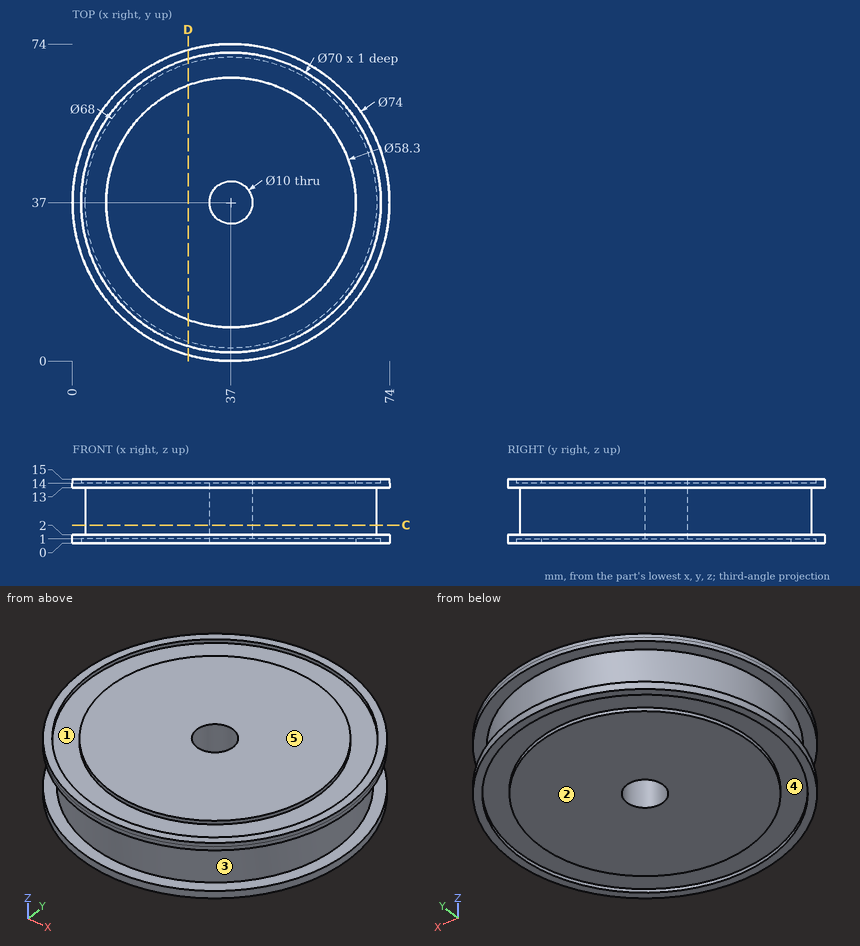
The figure shows three views and two pictorial views of one solid part (mm, origin at its lowest corner). Answer the questions. A direction names the side the tool comes from. Round coordinates to 2 decimals unless told otherwise and drop trailing zeros. Order: outer loops, then holes, each group sorted by start corner. A loop starts at its lowest first (then second) coordinate and runs counter-clockwise, first axis right, second up. Notation, with made-up numbers: M 4,73.5 L 54,73.5 A16 ccw 54,78.5 Z; hole C -22,39.25 d8. An arc over 180 degrees is marked long. Put each result on its own line as item: value. Start each with the question number.
Q1. Section D-D, the plane x = 27 is taken. Write down the section's boundary in (y, z), and give its area (3 significant figures).
Q2. For a pull along X with two mould halves and no side action, classify the marked faces 1, 2 and 3 as pulls with the +X half, pulls with the -X half, needs draft (parallel to the pull), parting line crosses it, or undercut.
Q3. Straight lines are drawn through the part: L1, parallel to Y at x = 37, z = 0.65; L2, parallel to Y at x = 37, z = 11; L3, parallel to Z at x = 67, y = 17. For each, find the intervals that lie inside material, in ascending order. Write a range as [from, to].
Q4. Flat-ended cylindrical pins translate along their axes: pin 1 (1.5 mm diameter, centred on x = 8.5, z = 6.5, fed in from -Y); pin 2 (2 mm diameter, centred on x = 20.5, z = 4.5, fed in from -Y); pin 3 (9 mm diameter, centred on x = 37, y = 37, fed in from +Z); pin 4 (3 mm diameter, centred on y = 36, z = 6, fed in from -X). Find the tip coordinate at first contact, or state that the pin passes through.
Q5. A tool of negligible diameter and unlimited length cuts with its end or side. For the marked faces 4 and 5, from which of +Z, -Z, +X, -X, +Y, -Y can it reach the whole face along a straight path? Write none if from no direction.
Q6. Section C-C, the plane z = 4.25 is taken. Write down the section's boundary in (x, y), and give its area (3 significant figures).
Findings below:
1. outline: M 1.38,0 L 3.46,0 L 3.46,1 L 9.62,1 L 9.62,0 L 64.38,0 L 64.38,1 L 70.54,1 L 70.54,0 L 72.62,0 L 72.62,2 L 69.5,2 L 69.5,13 L 72.62,13 L 72.62,15 L 70.54,15 L 70.54,14 L 64.38,14 L 64.38,15 L 9.62,15 L 9.62,14 L 3.46,14 L 3.46,15 L 1.38,15 L 1.38,13 L 4.5,13 L 4.5,2 L 1.38,2 Z
1. area: 975 mm^2
2. face 1: undercut
2. face 2: needs draft
2. face 3: parting line crosses it
3. L1: y = [0, 2], [7.85, 32], [42, 66.15], [72, 74]
3. L2: y = [3, 32], [42, 71]
3. L3: z = [0, 2], [13, 15]
4. pin 1: stops at y = 17.35
4. pin 2: stops at y = 6.74
4. pin 3: passes through
4. pin 4: stops at x = 3
5. face 4: -Z
5. face 5: +Z, +X, -X, +Y, -Y
6. outline: C 37,37 d68; hole C 37,37 d10
6. area: 3,550 mm^2
